Job drawing, mm, ordinate dimensions from the low corner. One solid piece. Give positions to 0.01 mm unless a question says otherwise; leave off trailing zeros. Write each loop counter-clockwise with the first axis right and the second up, starting at its lowest first coordinate (ties: lowest second). Pieces come first, ordered by that corner, then holes. Notation, with made-up numbers: (-28, 55) - (10, 55) arc R12 ccw to (10, 62) - close; hole circle Ø5 at (17, -37.5). An arc over 180 degrees is marked (long way). Use a Markdown table: item, result. Add a question column.
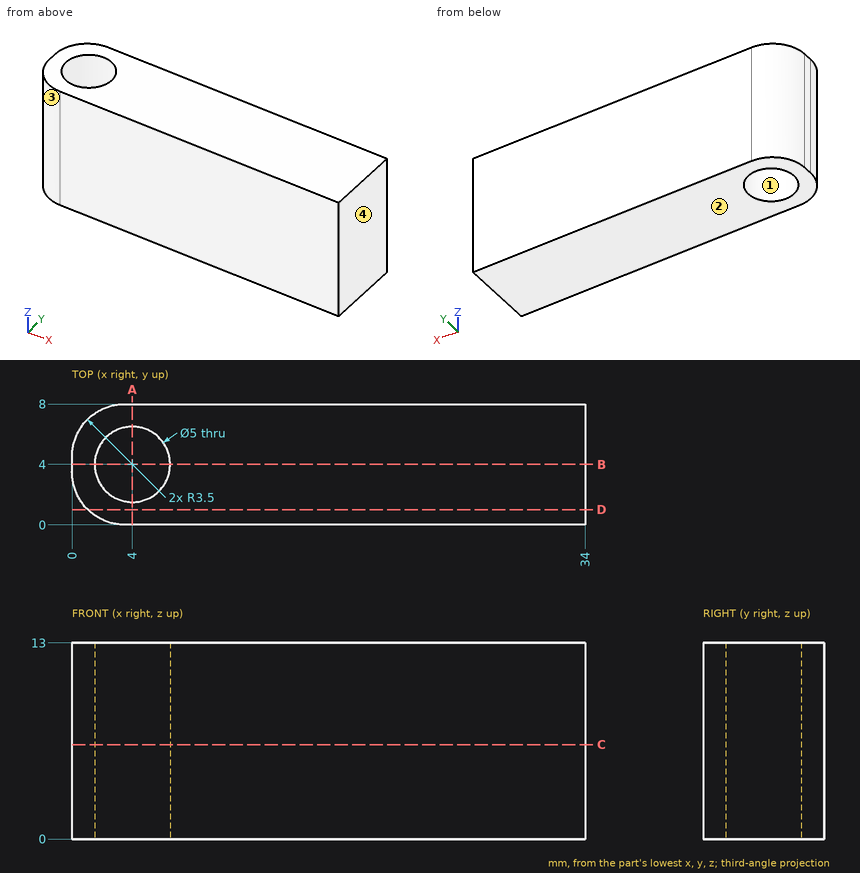
(1) Two-plate mould, pull along X, no slides. Class the marked faces 1, 2, 3 and 4: +X half, -X half, draft (parallel to the pull), parting line (faces both ways), or undercut.
(2) Flat gauge pin, fed straight in: pin 1 (4 mm diameter, centred on x = 4, y = 4, fed in from +Z). Where does the tip first touch, or does it go through?
(3) Band-saw the part on C-C (z = 6.25). Write the cut outline in (x, y), then the cut area to 3 significant figures.
(4) Probe probe 1 along Y at (x, z) = (4, 9); probe 2 along X at (y, z) = (5.5, 2.5); probe 3 along Y at (x, z) = (6, 3.75). List the from-to ranges inside material, lowest first. Write a range as [from, to].
(5) Band-saw the part on B-B (y = 4). Write the cut outline in (x, z), then the cut area to 3 significant figures.
(6) Band-saw the part on A-A (x = 4). Write the cut outline in (y, z).
(7) Band-saw the part on D-D (y = 1). Write the cut outline in (x, z).
Model answer:
| question | item | result |
|---|---|---|
| 1 | face 1 | undercut |
| 1 | face 2 | draft |
| 1 | face 3 | -X half |
| 1 | face 4 | +X half |
| 2 | pin 1 | passes through |
| 3 | outline | (0, 3.5) arc R3.5 ccw to (3.5, 0) - (34, 0) - (34, 8) - (3.5, 8) arc R3.5 ccw to (0, 4.5) - close; hole circle Ø5 at (4, 4) |
| 3 | area | 247 mm^2 |
| 4 | probe 1 | y = [0, 1.5], [6.5, 8] |
| 4 | probe 2 | x = [0.15, 2], [6, 34] |
| 4 | probe 3 | y = [0, 2.5], [5.5, 8] |
| 5 | outline | (0, 0) - (1.5, 0) - (1.5, 13) - (0, 13) - close; (6.5, 0) - (34, 0) - (34, 13) - (6.5, 13) - close |
| 5 | area | 377 mm^2 |
| 6 | outline | (0, 0) - (1.5, 0) - (1.5, 13) - (0, 13) - close; (6.5, 0) - (8, 0) - (8, 13) - (6.5, 13) - close |
| 7 | outline | (1.05, 0) - (34, 0) - (34, 13) - (1.05, 13) - close |
